Design review of the part built by this model. Coordinates are the model's own, in mm. A direction names the side the tool comes from. Round coordinates to 2 decimals unless told otherwise and drop trailing zeros. Order: outer loops, then holes, each group sorted by start corner. A loop starts at its lowest first (then second) coordinate and runs counter-clockwise, first axis right, second up. Notation, with made-up numbers: (34.25, 27.25) - (49.25, 27.25) arc R26 ccw to (49.25, 60.25) - close; hole circle Ø3 at (-29.75, 23). An arc over 180 degrees is marked (long way). Use CSV: the item, a comma, the result in double quotes.
from build123d import *

# Parameters (mm, degrees)
SKETCH4_W           = 108.585
SKETCH4_H           = 44.45
SKETCH4_W_2         = 98.425
SKETCH4_H_2         = 28.9052
BOSS_EXTRUDE2_DEPTH = 12.7
SKETCH5_W           = 108.585
SKETCH5_H           = 44.45
BOSS_EXTRUDE3_DEPTH = 3.556
SKETCH6_W           = 100.965
SKETCH6_H           = 44.45
SKETCH6_W_2         = 90.805
SKETCH6_H_2         = 29.0576
BOSS_EXTRUDE4_DEPTH = 12.7
BOSS_EXTRUDE6_DEPTH = 7.6962
BOSS_EXTRUDE7_DEPTH = 7.6962
FILLET1_R           = 2.54


with BuildPart() as part:
    # Sketch4 → Boss-Extrude2 (new body)
    with BuildSketch(Plane(origin=(0, 0, 0), x_dir=(0, 0, -1), z_dir=(1, 0, 0))):
        with Locations((49.2125, 14.4526)):
            Rectangle(SKETCH4_W, SKETCH4_H)
        with Locations((49.2125, 14.4526)):
            Rectangle(SKETCH4_W_2, SKETCH4_H_2, mode=Mode.SUBTRACT)
    extrude(amount=BOSS_EXTRUDE2_DEPTH)

    # Sketch5 → Boss-Extrude3 (add)
    with BuildSketch(Plane.ZY):
        with Locations((-49.2125, 14.4526)):
            Rectangle(SKETCH5_W, SKETCH5_H)
    extrude(amount=BOSS_EXTRUDE3_DEPTH)

    # Sketch6 → Boss-Extrude4 (add)
    with BuildSketch(Plane.ZY.offset(3.556)):
        with Locations((-45.4025, 14.4526)):
            Rectangle(SKETCH6_W, SKETCH6_H)
        with Locations((-45.4025, 14.4526)):
            Rectangle(SKETCH6_W_2, SKETCH6_H_2, mode=Mode.SUBTRACT)
    extrude(amount=BOSS_EXTRUDE4_DEPTH)

    # Sketch7 → Boss-Extrude6 (add)
    with BuildSketch(Plane(origin=(0, 36.6776, 0), x_dir=(1, 0, 0), z_dir=(0, 1, 0))):
        Polygon((-3.556, 103.505), (-3.556, 95.885), (-16.256, 95.885), align=None)
    extrude(amount=-BOSS_EXTRUDE6_DEPTH)

    # Sketch8 → Boss-Extrude7 (add)
    with BuildSketch(Plane.XZ.offset(7.7724)):
        Polygon((-3.556, -103.505), (-3.556, -95.885), (-16.256, -95.885), align=None)
    extrude(amount=-BOSS_EXTRUDE7_DEPTH)

    # Fillet1
    fillet1_edges = [part.edges().sort_by_distance(p)[0] for p in [
        (-3.556, 14.4526, -95.885),
        (-9.906, 28.9814, -95.885),
        (-3.556, 28.9814, -99.695),
        (-3.556, -0.0762, -99.695),
        (-9.906, -0.0762, -95.885),
    ]]
    fillet(fillet1_edges, radius=FILLET1_R)


solid = part.part
1) We need section B-B (y = 20). Give the boundary of the cut face in (x, z) (3 decimals).
Data:
outline,"(-16.256, -95.885) - (-6.096, -95.885) arc R2.54 cw to (-3.556, -98.425) - (-3.556, -103.505) - (12.7, -103.505) - (12.7, -98.425) - (0, -98.425) - (0, 0) - (12.7, 0) - (12.7, 5.08) - (-16.256, 5.08) - (-16.256, 0) - (-3.556, 0) - (-3.556, -90.805) - (-16.256, -90.805) - close"
2) We need section A-A (x = 8.25). Give the boundary of the cut face in (y, z) (3 decimals).
Data:
outline,"(-7.772, -103.505) - (36.678, -103.505) - (36.678, 5.08) - (-7.772, 5.08) - close; hole (0, -98.425) - (28.905, -98.425) - (28.905, 0) - (0, 0) - close"
3) We need section C-C (z = -33). Give the boundary of the cut face in (x, y).
Data:
outline,"(-16.26, -7.77) - (12.7, -7.77) - (12.7, 0) - (0, 0) - (0, 28.91) - (12.7, 28.91) - (12.7, 36.68) - (-16.26, 36.68) - (-16.26, 28.98) - (-3.56, 28.98) - (-3.56, -0.08) - (-16.26, -0.08) - close"
4) We need section D-D (y = 31). Give the boundary of the cut face in (x, z) (3 decimals).
Data:
outline,"(-16.256, -95.885) - (-3.556, -103.505) - (12.7, -103.505) - (12.7, 5.08) - (-16.256, 5.08) - close"
5) To check wall thickness, follow L1, parallel to Y at x = -5.5, z = -47.5; L2, parallel to Z at x = 2.5, y = 18 (3 decimals); L3, parallel to Y at x = 5.75, z = -15.5. State the ranges of each line that lie inside material, in increasing order. Write a range as from..to.
Data:
L1,"y = -7.77..-0.08, 28.98..36.68"
L2,"z = -103.505..-98.425, 0..5.08"
L3,"y = -7.77..0, 28.91..36.68"
6) For faces 1 (the face through (6, 0, -49)), 2 (the face through (-10.118, 0.648, -96.649)), 3 (the face through (-10, -0.076, -46)), 4 (the face through (-9.995, -3.863, -99.642)), 5 (the face through (-16.256, 30, -57)), list the 3-axis set-ups (+Z, -Z, +X, -X, +Y, -Y) from which the entire face can be reached by the end or side of a thin tool; tool diameter is ignored.
Data:
face 1,"+X"
face 2,"-Z, -X"
face 3,"-X"
face 4,"-Z, -X, +Y, -Y"
face 5,"+Z, -Z, -X, +Y, -Y"
7) Insertion check: pin 1 Ø3 at (y, z) = (26.5, -33) entering from +X; pin 2 Ø6 at (y, z) = (3, -58) entering from -X; pin 3 Ø4 at (x, y) = (-7.5, 11) entering from -Z. Each pin has a flat end and moves straight along its axis. Give the tip position at first contact, or say it passes through.
Data:
pin 1,"stops at x = 0"
pin 2,"stops at x = -3.56"
pin 3,"stops at z = -95.96"
8) The part is to be moulded in two halves that separate along Y. For faces 6 (the face through (-2, 36.678, -50)), 7 (the face through (-3.556, 15, -101)), 8 (the face through (5, 14, -103.505)), say which applies: +Y half, -Y half, draft (parallel to the pull), parting line (faces both ways), or undercut.
Data:
face 6,"+Y half"
face 7,"undercut"
face 8,"draft"
